Input: dimensioned drawing with shaded views. Units: mm. Origin: part minimum x, y, z. Round coordinates to 2 decimals unless told otherwise and drop trailing zeros. Order: outer loops, then holes, each group sorted by start corner. A loop starts at its lowest first (then second) coordinate and runs counter-clockwise, first axis right, second up.
Item 1: Cut plane B-B on x = 110. Output: boundary loops of the cut face in (y, z), then the cut area to 3 significant figures.
Item 2: Line query: L1, parallel to X at y = 3.25, z = 65. Output: solid intervals per line, ascending.
Item 3: Cut plane A-A on z = 65. Output: boundary loops of the cut face in (x, y).
Item 4: First-contact query: pin 1 (3.5 mm diameter, centred on x = 50, z = 65, fed in from -Y). Flat tip, straight axial feed; report the tip coordinate or a pass-through.
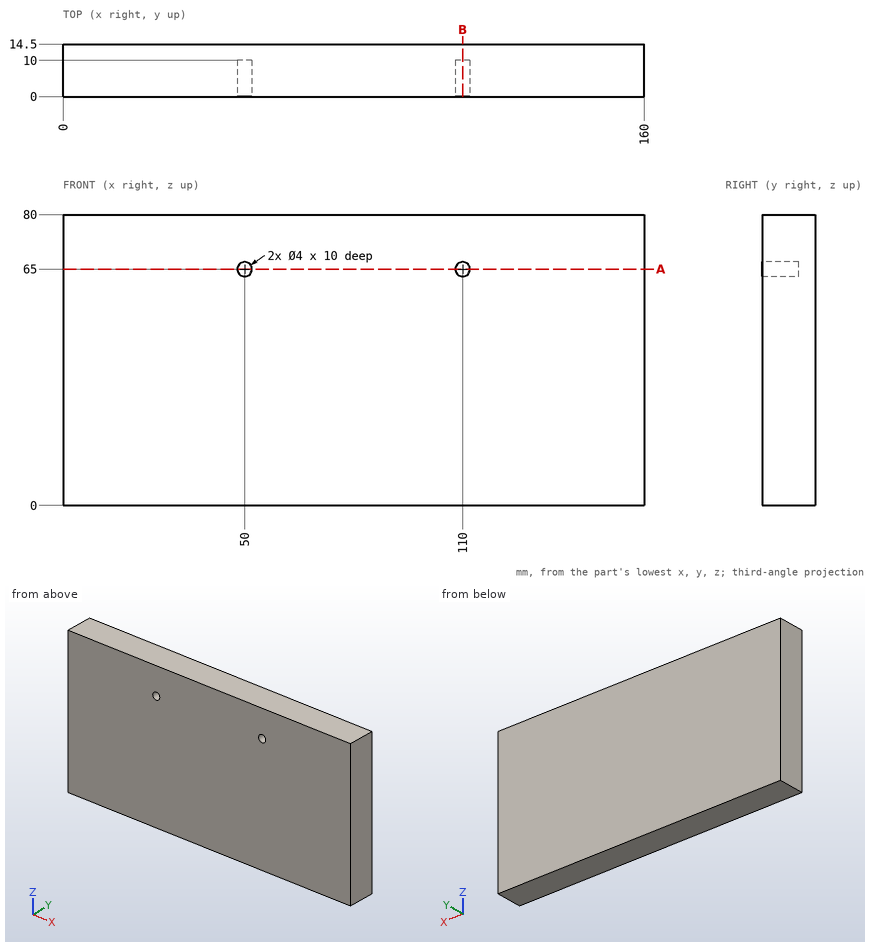
From the geometry:
1. outline: (0, 0) - (14.5, 0) - (14.5, 80) - (0, 80) - (0, 67) - (10, 67) - (10, 63) - (0, 63) - close
1. area: 1,120 mm2
2. L1: x = 0 to 48, 52 to 108, 112 to 160
3. outline: (0, 0) - (48, 0) - (48, 10) - (52, 10) - (52, 0) - (108, 0) - (108, 10) - (112, 10) - (112, 0) - (160, 0) - (160, 14.5) - (0, 14.5) - close
4. pin 1: stops at y = 10
